Autodesk Inventor part; units mm, degrees
sketch "Sketch1" plane through (0, 0, 0) normal (0, 0, 1) x (1, 0, 0)
  line L0 (0, 2.8582) -> (0, -2.8582) construction
  line L1 (-5.7775, 0) -> (5.7775, 0) construction
  point P0 (0, 0)
  point P1 (0, 0)
sketch "Sketch2" plane through (0, 0, 0) normal (0, 0, 1) x (1, 0, 0)
  line L0 (2.4826, 4.3) -> (4.9652, 0)
  line L1 (4.9652, 0) -> (2.4826, -4.3)
  line L2 (2.4826, -4.3) -> (-2.4826, -4.3)
  line L3 (-2.4826, -4.3) -> (-4.9652, 0)
  line L4 (-4.9652, 0) -> (-2.4826, 4.3)
  line L5 (-2.4826, 4.3) -> (2.4826, 4.3)
  line L6 (-7.5, 7.5) -> (7.5, 7.5)
  line L7 (7.5, 7.5) -> (7.5, -7.5)
  line L8 (7.5, -7.5) -> (-7.5, -7.5)
  line L9 (-7.5, -7.5) -> (-7.5, 7.5)
  line L10 (-7.5, 7.5) -> (7.5, -7.5) construction
  line L11 (7.5, 7.5) -> (-7.5, -7.5) construction
  point P0 (0, 0)
  point P1 (0, 0)
  dimension "d0" = 8.6
  dimension "d1" = 15
  dimension "d2" = 15
extrude "Extrusion1" add sketch "Sketch2" along normal blind 5
chamfer "Chamfer1" distance 3 angle 45 1 edges at (7.5, 7.5, 2.5)
sketch "Sketch3" plane through (-7.5, -7.5, 0) normal (-1, 0, 0) x (0, 0, 1)
  line L0 (0, 15) -> (5, 15)
  line L1 (5, 15) -> (5, 10)
  line L2 (5, 10) -> (0, 10)
  line L3 (0, 10) -> (0, 15)
  point P0 (0, 7.5)
  dimension "d8" = 5
  dimension "d9" = 5
extrude "Extrusion2" add sketch "Sketch3" along normal blind 5
sketch "Sketch4" plane through (-7.5, -7.5, 0) normal (0, -1, 0) x (1, 0, 0)
  line L0 (15, 0) -> (15, 5)
  line L1 (15, 5) -> (10, 5)
  line L2 (10, 5) -> (10, 0)
  line L3 (10, 0) -> (15, 0)
  line L4 (15, 0) -> (15, 5)
  point P0 (7.5, 0)
  dimension "d12" = 5
  dimension "d13" = 5
extrude "Extrusion3" add sketch "Sketch4" along normal blind 5
properties part number "bevestiging deksel" material "S235"
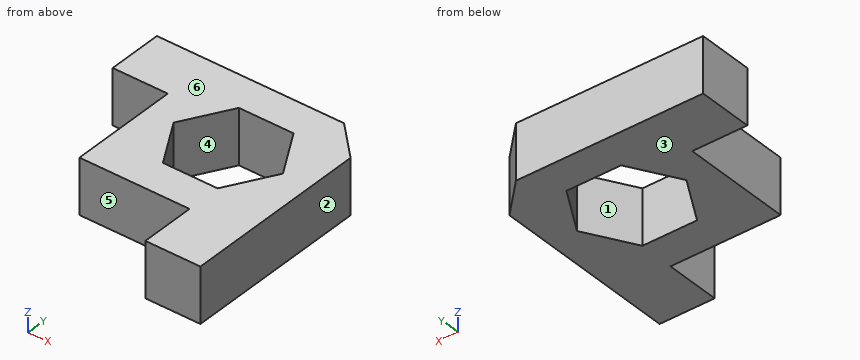
CAD build for the part. Positions are in the model's coordinates, mm. Face numbers are marked on the shaded views. A direction names the side the tool comes from. Give positions to 0.01 mm unless a question says otherwise; leave off trailing zeros. Order: outer loops, then holes, each group sorted by start corner. A loop starts at its lowest first (then second) coordinate and runs counter-clockwise, first axis right, second up. Notation, with made-up numbers: M 36,13 L 91,13 A33 cw 91,51 Z; hole C 24,61.5 d8. An arc over 180 degrees is marked long. Put each result on its own line as item: value. Start each with the question number.
(1) Saw through at B-B, the plane y = -3.25. Write the cut outline in (x, z), then the cut area to 3 significant figures.
(2) Drill centre lines: line 1 along Y through (x, z) = (1.5, 2.15); line 2 along Y through (x, z) = (-4, 3.8); line 3 along X through (y, z) = (2, 2.85). Where is each one in solid material? Low to high.
(3) Saw through at C-C, the plane z = 4.55. Write the cut outline in (x, y).
(4) Saw through at A-A, the plane x = 1.75. Write the cut outline in (y, z).
(5) Mould opens along X. For the marked faces 1, 2 and 3 say: +X half, -X half, draft (parallel to the pull), parting line (faces both ways), or undercut.
(6) Which spindle directions (+Z, -Z, +X, -X, +Y, -Y) get a long thin tool onto all of the face, cutting with end or side? Do the marked faces 4, 5 and 6. Say none if no direction does.
(7) Saw through at D-D, the plane y = -5.25. Write the cut outline in (x, z).
(8) Flat gauge pins, fed straight in: pin 1 Ø4 at (x, y) = (-10, -8.5) entering from -Z; pin 2 Ø1 at (x, z) = (-9, 4.5) entering from -Y; pin 3 Ø1.5 at (x, y) = (-4, -1) entering from -Z; pin 4 Ø2 at (y, z) = (0.5, 4) entering from -X. Where does each tip first touch, or does it go through?
Check result:
1. outline: M -7.5,0 L -3.09,0 L -3.09,5 L -7.5,5 Z; M 3.09,0 L 7.5,0 L 7.5,5 L 3.09,5 Z
1. area: 44.1 mm2
2. line 1: y = -7.5 to -4.3, 4.3 to 7.5
2. line 2: y = -7.5 to -1.67, 1.67 to 7.5
2. line 3: x = -7.5 to -3.81, 3.81 to 7.5
3. outline: M -12.5,2.5 L -7.5,2.5 L -7.5,-7.5 L 2.5,-7.5 L 2.5,-12.5 L 7.5,-12.5 L 7.5,4.5 L 4.5,7.5 L -12.5,7.5 Z; hole M -4.97,0 L -2.48,-4.3 L 2.48,-4.3 L 4.97,0 L 2.48,4.3 L -2.48,4.3 Z
4. outline: M -7.5,0 L -4.3,0 L -4.3,5 L -7.5,5 Z; M 4.3,0 L 7.5,0 L 7.5,5 L 4.3,5 Z
5. face 1: undercut
5. face 2: +X half
5. face 3: draft
6. face 4: +Z, -Z
6. face 5: +Z, -Z, -X, -Y
6. face 6: +Z, +X, -X, +Y, -Y
7. outline: M -7.5,0 L 7.5,0 L 7.5,5 L -7.5,5 Z
8. pin 1: passes through
8. pin 2: stops at y = 2.5
8. pin 3: stops at z = 0
8. pin 4: stops at x = -7.5
